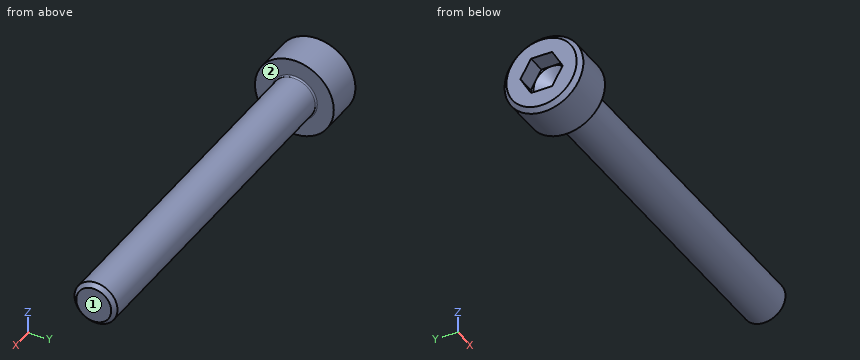
```python
from build123d import *

# Parameters (mm, degrees)
FILLET1_R   = 0.1
HEX_2_DEPTH = 1.3


with BuildPart() as part:
    # BodySke → Base-Revolve (revolve)
    with BuildSketch(Plane.XY):
        Polygon((0, 0), (0, 2.45), (0.3, 2.75), (3, 2.75), (3, 1.5), (27.7195, 1.5), (28, 1.2195), (28, 0), align=None)
    revolve(axis=Axis((-31.75, 0, 0), (1, 0, 0)))

    # Fillet1
    fillet1_edges = [part.edges().sort_by_distance(p)[0] for p in [
        (3, -1.5, 0),
    ]]
    fillet(fillet1_edges, radius=FILLET1_R)

    # Sketch2 → Hex-PreBroach (revolve, cut)
    with BuildSketch(Plane.XY):
        Polygon((0, 1.28), (1.3, 1.28), (2.039008345, 0), (0, 0), align=None)
    revolve(axis=Axis((0, 0, 0), (1, 0, 0)), mode=Mode.SUBTRACT)

    # Sketch3 → Hex 2 (cut)
    with BuildSketch(Plane(origin=(0, 0, 0), x_dir=(0, 0.5, 0.866025404), z_dir=(-1, 0, 0))):
        Polygon((0.739008345, 1.28), (-0.739008345, 1.28), (-1.478016689, 0), (-0.739008345, -1.28), (0.739008345, -1.28), (1.478016689, 0), align=None)
    extrude(amount=-HEX_2_DEPTH, mode=Mode.SUBTRACT)


solid = part.part
```
Model file for the job. Use its own axes, mm. Face numbers are marked on the shaded views. A direction names the side the tool comes from. Round coordinates to 2 decimals unless told otherwise and drop trailing zeros. Use CSV: the item, a comma, the result in double quotes. Start each with the question number.
Item 1: Pin check, flat tip, straight feed: P1, Ø2, axis at x = 15, y = -1, coming from the +Z side. Stop position of the tip, or through.
Item 2: Tool access for the marked faces 1 and 2: list every direction of +Z, -Z, +X, -X, +Y, -Y with a clear straight run to the whole face (end or side of a thin tool).
Item 3: Drill centre lines: L1, parallel to X at y = -0.3, z = 2.2; L2, parallel to Z at x = 21.5, y = 0.1; L3, parallel to Y at x = 6.5, z = -0.6. Where is each one in solid material? Low to high. Write a range as [from, to].
Checked values:
1,P1,"stops at z = 1.5"
2,face 1,"+Z, -Z, +X, +Y, -Y"
2,face 2,"+X"
3,L1,"x = [0, 3]"
3,L2,"z = [-1.5, 1.5]"
3,L3,"y = [-1.37, 1.37]"
